```python
from build123d import *

# Parameters (mm, degrees)
SKETCH1_W            = 106
SKETCH1_H            = 78
BOSS_EXTRUDE1_DEPTH  = 50
HOLEWZD1_D           = 4.5
HOLEWZD2_D           = 4.2
HOLEWZD2_DEPTH       = 30
HOLEWZD4_D           = 20
HOLEWZD4_DEPTH       = 20
HOLEWZD4_CSINK_D     = 22
HOLEWZD4_CSINK_ANGLE = 90
HOLEWZD5_AT_2_COUNT  = 2
HOLEWZD5_AT_2_PITCH  = 28
HOLEWZD5_AT_3_COUNT  = 2
HOLEWZD5_AT_3_PITCH  = 56
HOLEWZD5_AT_4_COUNT  = 2
HOLEWZD5_AT_4_PITCH  = 62.60990337
HOLEWZD6_D           = 16
HOLEWZD6_DEPTH       = 45
HOLEWZD6_CSINK_D     = 19
HOLEWZD6_CSINK_ANGLE = 90
CHAMFER1_SIZE        = 1.5
FILLET1_R            = 5


# Read off the part's stored shape, not the designer's step: HoleWzd3
with BuildPart() as part:
    # Sketch1 → Boss-Extrude1 (new body)
    with BuildSketch(Plane(origin=(0, 0, 0), x_dir=(-1, 0, 0), z_dir=(0, 0, -1))):
        with Locations((-42, 28)):
            Rectangle(SKETCH1_W, SKETCH1_H)
    extrude(amount=-BOSS_EXTRUDE1_DEPTH)

    # HoleWzd1 (through all)
    with Locations(Plane.XY.offset(50)):
        with Locations((14, 59.5), (70, -3.5), (14, -3.5), (70, 59.5)):
            Hole(HOLEWZD1_D / 2)

    # HoleWzd2
    with Locations(Plane(origin=(0, 67, 0), x_dir=(1, 0, 0), z_dir=(0, 1, 0))):
        with Locations((42, -25)):
            Hole(HOLEWZD2_D / 2, depth=HOLEWZD2_DEPTH)

    # HoleWzd3 outline → HoleWzd3 (revolve, cut)
    with BuildSketch(Plane(origin=(42, 50, 0), x_dir=(1, 0, 0), z_dir=(0, -1, 0))):
        Polygon((0, 14.648924226), (1.25, 15.4), (1.25, 23.312743137), (0, 23.312743137), align=None)
    revolve(axis=Axis((42, 50, 0), (0, 0, 1)), mode=Mode.SUBTRACT)

    # HoleWzd4
    with Locations(Plane(origin=(0, 0, 0), x_dir=(-1, 0, 0), z_dir=(0, 0, -1))):
        with Locations((-42, 14), (-42, 42)):
            CounterSinkHole(HOLEWZD4_D / 2, HOLEWZD4_CSINK_D / 2, depth=HOLEWZD4_DEPTH, counter_sink_angle=HOLEWZD4_CSINK_ANGLE)

    # Sketch9 → HoleWzd5 (revolve, cut)
    with BuildSketch(Plane(origin=(70, 42, 0), x_dir=(0, 1, 0), z_dir=(1, 0, 0))):
        Polygon((0, 0), (0, 50), (2.25, 50), (2.25, 20), (10, 20), (10, 1), (11, 0), align=None)
    holewzd5 = revolve(axis=Axis((70, 42, -6.35), (0, 0, 1)), mode=Mode.SUBTRACT)

    # HoleWzd5 at 2: HoleWzd5 ×2
    with Locations(*[(0, -i * HOLEWZD5_AT_2_PITCH, 0) for i in range(1, HOLEWZD5_AT_2_COUNT)]):
        add(holewzd5, mode=Mode.SUBTRACT)

    # HoleWzd5 at 3: HoleWzd5 ×2
    with Locations(*[(-i * HOLEWZD5_AT_3_PITCH, 0, 0) for i in range(1, HOLEWZD5_AT_3_COUNT)]):
        add(holewzd5, mode=Mode.SUBTRACT)

    # HoleWzd5 at 4: HoleWzd5 ×2
    with Locations(*[Vector(-0.894427190999916, -0.447213595499958, 0) * (i * HOLEWZD5_AT_4_PITCH) for i in range(1, HOLEWZD5_AT_4_COUNT)]):
        add(holewzd5, mode=Mode.SUBTRACT)

    # HoleWzd6
    with Locations(Plane(origin=(0, 0, 0), x_dir=(-1, 0, 0), z_dir=(0, 0, -1))):
        with Locations((-84, 56), (-84, 28), (-56, 56), (-56, 0), (-84, 0), (-28, 28), (-28, 56), (-56, 28), (-28, 0), (0, 28), (0, 0), (0, 56)):
            CounterSinkHole(HOLEWZD6_D / 2, HOLEWZD6_CSINK_D / 2, depth=HOLEWZD6_DEPTH, counter_sink_angle=HOLEWZD6_CSINK_ANGLE)

    # Chamfer1
    chamfer1_edges = [part.edges().sort_by_distance(p)[0] for p in [
        (48, 0, 45),
    ]]
    chamfer(chamfer1_edges, length=CHAMFER1_SIZE)

    # Fillet1
    fillet1_edges = [part.edges().sort_by_distance(p)[0] for p in [
        (95, -11, 25),
        (95, 67, 25),
        (-11, 67, 25),
        (-11, -11, 25),
    ]]
    fillet(fillet1_edges, radius=FILLET1_R)


solid = part.part
```
Could you check a few things on this model? Use its own coordinates, in mm. A direction names the side the tool comes from. Coordinates: 2 decimals unless noted, no trailing zeros. Use a Markdown table: item, result. Add a question column.
Q1. We'd pull the mould along Y, two halves only. Please class faces 1 (the cylindrical face through (-9, -10, 25)), 2 (the flat face through (14, 28, 0)), 3 (the cylindrical face through (72.196, 13.512, 34.79)), 4 (the flat face through (0, 0, 45)): pulls with the +Y half, pulls with the -Y half, needs draft (parallel to the pull), parting line crosses it, or undercut.
Q2. I want a section at A-A on y = 14. Give the number of separate pieces and of enclosed holes in the cut face, then the cut area to 3 significant figures.
Q3. If I drill on L1, parallel to Y at x = 84, z = 27; L2, parallel to X at y = 56, z = 15; L3, parallel to Y at x = 14, z = 36, over which ranges is the centre line in solid material (lowest first)?
Q4. I'm going to push flat-ended pins straight in: pin 1 (5 mm diameter, centred on x = 80.5, y = 27.5, fed in from -Z); pin 2 (14.5 mm diameter, centred on x = 56, y = 0, fed in from -Z). Where does each tip first touch, or does it pass through?
Q5. Which directions (+Z, -Z, +X, -X, +Y, -Y) give clear straight access to the entire face, cutting with the end or side of a thin tool? Please do faces 5 (the flat face through (42, 37, 25)), 6 (the cylindrical face through (79.76, 11.83, 10.37)), 7 (the flat face through (70, 28, 0)).
Checked values:
| question | item | result |
|---|---|---|
| 1 | face 1 | pulls with the -Y half |
| 1 | face 2 | needs draft |
| 1 | face 3 | undercut |
| 1 | face 4 | undercut |
| 2 | separate pieces | 3 |
| 2 | enclosed holes | 0 |
| 2 | area | 3,830 mm² |
| 3 | L1 | -11 to -8, 8 to 20, 36 to 48, 64 to 67 |
| 3 | L2 | -11 to -8, 8 to 20, 36 to 48, 64 to 76, 92 to 95 |
| 3 | L3 | -11 to -5.75, -1.25 to 11.75, 16.25 to 39.75, 44.25 to 57.25, 61.75 to 67 |
| 4 | pin 1 | z = 45 |
| 4 | pin 2 | z = 44.25 |
| 5 | face 5 | +Y |
| 5 | face 6 | -Z |
| 5 | face 7 | -Z, +X, -X, +Y, -Y |
